from build123d import *

# Parameters (mm, degrees)
SKETCH1_R           = 28.575
BOSS_EXTRUDE1_DEPTH = 10.16
SKETCH2_R           = 16.51
CUT_EXTRUDE1_DEPTH  = 42.66877548
SKETCH3_R           = 22.86
CUT_EXTRUDE2_DEPTH  = 8.255
SKETCH4_W           = 88.915115744
SKETCH4_H           = 51.352535237
CUT_EXTRUDE3_DEPTH  = 42.66877548
CUT_EXTRUDE4_REACH  = 43.669
SKETCH6_R           = 1.778


with BuildPart() as part:
    # Sketch1 → Boss-Extrude1 (new body)
    with BuildSketch(Plane(origin=(0, 0, 0), x_dir=(1, 0, 0), z_dir=(0, 1, 0))):
        with Locations(Location((0, 0, 0), (0, 0, 270))):
            Circle(SKETCH1_R)
    extrude(amount=BOSS_EXTRUDE1_DEPTH)

    # Sketch2 → Cut-Extrude1 (cut, through all)
    with BuildSketch(Plane.XZ):
        with Locations(Location((0, 0, 0), (0, 0, 270))):
            Circle(SKETCH2_R)
    extrude(amount=-CUT_EXTRUDE1_DEPTH, mode=Mode.SUBTRACT)

    # Sketch3 → Cut-Extrude2 (cut)
    with BuildSketch(Plane.XZ):
        with Locations(Location((0, 0, 0), (0, 0, 270))):
            Circle(SKETCH3_R)
    extrude(amount=-CUT_EXTRUDE2_DEPTH, mode=Mode.SUBTRACT)

    # Sketch4 → Cut-Extrude3 (cut, through all)
    with BuildSketch(Plane(origin=(0, 10.16, 0), x_dir=(1, 0, 0), z_dir=(0, 1, 0))):
        with Locations((4.883047594, -25.676267619)):
            Rectangle(SKETCH4_W, SKETCH4_H)
    extrude(amount=-CUT_EXTRUDE3_DEPTH, mode=Mode.SUBTRACT)

    # Sketch6 → Cut-Extrude4 (cut, up to next)
    with BuildSketch(Plane.XZ, mode=Mode.PRIVATE) as cut_extrude4_sk1:
        with Locations(Location((18.185018645, -18.185018645, 0), (0, 0, 270))):
            Circle(SKETCH6_R)
    cut_extrude4_tool1 = extrude(cut_extrude4_sk1.sketch, amount=-CUT_EXTRUDE4_REACH, mode=Mode.PRIVATE) & part.part
    # Sketch6 → Cut-Extrude4 (cut, up to next)
    with BuildSketch(Plane.XZ, mode=Mode.PRIVATE) as cut_extrude4_sk2:
        with Locations(Location((-18.185018645, -18.185018645, 0), (0, 0, 270))):
            Circle(SKETCH6_R)
    cut_extrude4_tool2 = extrude(cut_extrude4_sk2.sketch, amount=-CUT_EXTRUDE4_REACH, mode=Mode.PRIVATE) & part.part
    add(cut_extrude4_tool1.solids().sort_by_distance((18.185019, 0, -18.185019))[0], mode=Mode.SUBTRACT)
    add(cut_extrude4_tool2.solids().sort_by_distance((-18.185019, 0, -18.185019))[0], mode=Mode.SUBTRACT)


solid = part.part
Geometry check sheet. Reference: the model listing, model coordinates, mm. A direction names the side the tool comes from. Round coordinates to 2 decimals unless told otherwise and drop trailing zeros. Write each loop counter-clockwise with the first axis right and the second up, starting at its lowest first coordinate (ties: lowest second). Pieces come first, ordered by that corner, then holes. Notation, with made-up numbers: (32.25, 30) -> (80.25, 30) arc R10 ccw to (80.25, 40) -> close; hole circle Ø7 at (73, 61). An arc over 180 degrees is marked (long way). One line per item, written item: value. Start each with the question number.
(1) Access from +Z, -Z, +X, -X, +Y, -Y to the whole of each face (thin tool, end or side, straight path). Record for faces 5 (the cylindrical face through (-0.503, 4.07, -22.854)), 6 (the flat face through (-2, 0, -23)).
(2) Cross-section at C-C, the plane y = 0.75. Record the cut outline in (x, z) (3 decimals).
(3) Draft check along Z on faces 1 (the cylindrical face through (16.45, 5.01, -17.8)), 2 (the flat face through (0, 10.16, -18)), 3 (the cylindrical face through (-19.3, 5, -16.8)), 4 (the flat face through (-25, 6, 0)). Enter one of: +Z half, -Z half, draft (parallel to the pull), parting line (faces both ways), or undercut.
(4) Scan lines: line 1 (Y direction, x = 19, z = -3) (3 decimals); line 2 (X direction, y = 4.5, z = -7.25); line 3 (X direction, y = 8.5, z = -19.5). Record each from-to range of solid material in increasing order. Write a range as [from, to].
(5) Go/stop test with flat-tipped pins: pin 1 Ø1 at (x, y) = (-13.5, 8) entering from -Z; pin 2 Ø5 at (y, z) = (5.5, -17) entering from +X; pin 3 Ø1.5 at (x, y) = (5.5, 8) entering from +Z. Record where each tip stops, or that it passes through.
(6) Cross-section at A-A, the plane z = -7.75. Record the cut outline in (x, y) (3 decimals).
(7) Cross-section at B-B, the plane x = 0. Record the cut outline in (y, z) (3 decimals).
(8) Cross-section at D-D, the plane z = -22. Record the cut outline in (x, y) (3 decimals).
Answer:
1. face 5: +Z, -Y
1. face 6: +Z, -Z, +X, -X, -Y
2. outline: (-28.575, 0) arc R28.575 ccw to (28.575, 0) -> (22.86, 0) arc R22.86 cw to (-22.86, 0) -> close; hole circle Ø3.556 at (-18.185, -18.185); hole circle Ø3.556 at (18.185, -18.185)
3. face 1: undercut
3. face 2: draft
3. face 3: undercut
3. face 4: +Z half
4. line 1: [8.255, 10.16]
4. line 2: [-27.64, -21.68], [21.68, 27.64]
4. line 3: [-20.89, -19.38], [-16.99, 16.99], [19.38, 20.89]
5. pin 1: z = -25.45
5. pin 2: x = 24.62
5. pin 3: z = -15.3
6. outline: (-27.504, 0) -> (-21.506, 0) -> (-21.506, 8.255) -> (-14.578, 8.255) -> (-14.578, 10.16) -> (-27.504, 10.16) -> close; (14.578, 8.255) -> (21.506, 8.255) -> (21.506, 0) -> (27.504, 0) -> (27.504, 10.16) -> (14.578, 10.16) -> close
7. outline: (0, -28.575) -> (10.16, -28.575) -> (10.16, -16.51) -> (8.255, -16.51) -> (8.255, -22.86) -> (0, -22.86) -> close
8. outline: (-18.235, 0) -> (-6.211, 0) -> (-6.211, 8.255) -> (6.211, 8.255) -> (6.211, 0) -> (18.235, 0) -> (18.235, 10.16) -> (-18.235, 10.16) -> close
